For this review, take the finished solid that the model builds, in its own axes (mm). Give positions to 0.01 mm unless a question says otherwise; leave off trailing zeros. Order: outer loops, then holes, each group sorted by start corner. A loop starts at its lowest first (then second) coordinate and runs counter-clockwise, first axis right, second up. Notation, with made-up numbers: (67, 41.25) - (82, 41.25) arc R21 cw to (82, 74.25) - close; hole circle Ø5 at (30, 44). An arc over 180 degrees is marked (long way). Use a Markdown table: item, result. Add a question column.
1) Clearance check with flat-ended pins moving along their axes: P1, Ø1, axis at x = -7, y = -32, coming from the +Z side; P2, Ø2, axis at y = 135.5, z = -1.5, coming from the +X side; P3, Ø12, axis at x = 8.5, z = -3, coming from the -Y side. State where each tip first meets the part, or that it passes through.
2) Mouldability with a two-part tool opening along X and no side actions: class faces 1 (the face through (6.611, 355.763, -9.439)), 2 (the face through (-11.23, 362.34, -0.99)), 3 (the face through (-10.787, -5.153, -2.395)) as released by +X, released by -X, zero draft, split by the parting line, or undercut.
3) Wall thickness on L1, parallel to Z at x = 0, y = -139; L2, parallel to Z at x = 5, y = 68: over which ranges is each line inside the solid? List them lowest first.
4) We need section B-B on y = -167.5. Write out the cut boundary in (x, z), then the cut area to 3 significant figures.
5) We need section A-A on z = 0. Write out the cut boundary in (x, y), then the cut area to 3 significant figures.
```python
from build123d import *

# Parameters (mm, degrees)
SKETCH1_R           = 12.7
SKETCH1_R_2         = 11.05
BOSS_EXTRUDE1_DEPTH = 375
SKETCH2_R           = 13
CUT_EXTRUDE1_DEPTH  = 751.21502251
CUT_EXTRUDE2_START  = -12.606982135
CUT_EXTRUDE2_DEPTH  = 25.21396427


# Read off the part's stored shape, not the designer's step: Cut-Extrude2
with BuildPart() as part:
    # Sketch1 → Boss-Extrude1 (new, symmetric)
    with BuildSketch(Plane(origin=(0, 0, 0), x_dir=(1, 0, 0), z_dir=(0, 1, 0))):
        with Locations(Location((0, 0, 0), (0, 0, 270))):
            Circle(SKETCH1_R)
        with Locations(Location((0, 0, 0), (0, 0, 270))):
            Circle(SKETCH1_R_2, mode=Mode.SUBTRACT)
    extrude(amount=BOSS_EXTRUDE1_DEPTH, both=True)

    # Sketch2 → Cut-Extrude1 (cut, symmetric)
    with BuildSketch(Plane(origin=(0, -375, 0), x_dir=(0, 0, -1), z_dir=(0.707545129365096, 0.7066681610994865, 0))):
        Circle(SKETCH2_R)
    cut_extrude1 = extrude(amount=CUT_EXTRUDE1_DEPTH, both=True, mode=Mode.SUBTRACT)

    # Mirror1: Cut-Extrude1 across plane
    add(cut_extrude1.mirror(Plane.ZX), mode=Mode.SUBTRACT)

    # Cut-Extrude2 outline → Cut-Extrude2 (cut)
    with BuildSketch(Plane.XY.offset(CUT_EXTRUDE2_START)):
        Polygon((0, -373.584908653), (-1.534275545, -372.048729087), (-12.7, -360.869148077), (-14, -359.56753479), (-14, -374), (0, -374), align=None)
    cut_extrude2 = extrude(amount=CUT_EXTRUDE2_DEPTH, mode=Mode.SUBTRACT)

    # Mirror2: Cut-Extrude2 across plane
    add(cut_extrude2.mirror(Plane.ZX), mode=Mode.SUBTRACT)


solid = part.part
```
Checked values:
| question | item | result |
|---|---|---|
| 1 | P1 | z = 10.91 |
| 1 | P2 | x = 12.69 |
| 1 | P3 | y = -354.65 |
| 2 | face 1 | released by +X |
| 2 | face 2 | released by -X |
| 2 | face 3 | undercut |
| 3 | L1 | -12.7 to -11.05, 11.05 to 12.7 |
| 3 | L2 | -11.67 to -9.85, 9.85 to 11.67 |
| 4 | outline | circle Ø25.4 at (0, 0); hole circle Ø22.1 at (0, 0) |
| 4 | area | 123 mm² |
| 5 | outline | (-12.7, -360.87) - (-11.05, -362.52) - (-11.05, 362.52) - (-12.7, 360.87) - close; (11.05, -345.59) - (12.7, -343.94) - (12.7, 343.94) - (11.05, 345.59) - close |
| 5 | area | 2,330 mm² |
